```python
from build123d import *

# Parameters (mm, degrees)
SKETCH1_W           = 120
SKETCH1_H           = 92
SKETCH1_R           = 1.5
BOSS_EXTRUDE1_DEPTH = 1
SKETCH2_W           = 1
SKETCH2_H           = 92
BOSS_EXTRUDE2_DEPTH = 23
FILLET1_R           = 3
FILLET2_R           = 3
FILLET3_R           = 3


with BuildPart() as part:
    # Sketch1 → Boss-Extrude1 (new body)
    with BuildSketch(Plane.XY):
        Rectangle(SKETCH1_W, SKETCH1_H)
        with Locations((0, -32)):
            Circle(SKETCH1_R, mode=Mode.SUBTRACT)
        with Locations(Location((0, 32, 0), (0, 0, 180))):
            Circle(SKETCH1_R, mode=Mode.SUBTRACT)
    extrude(amount=BOSS_EXTRUDE1_DEPTH)

    # Sketch2 → Boss-Extrude2 (add)
    with BuildSketch(Plane.XY.offset(1)):
        with Locations((-59.5, 0)):
            Rectangle(SKETCH2_W, SKETCH2_H)
    boss_extrude2 = extrude(amount=BOSS_EXTRUDE2_DEPTH)

    # Fillet1
    fillet1_edges = [part.edges().sort_by_distance(p)[0] for p in [
        (-60, 0, 0),
    ]]
    fillet(fillet1_edges, radius=FILLET1_R)

    # Fillet2
    fillet2_edges = [part.edges().sort_by_distance(p)[0] for p in [
        (-59, 0, 1),
    ]]
    fillet(fillet2_edges, radius=FILLET2_R)

    # Mirror3: Boss-Extrude2 across plane
    add(boss_extrude2.mirror(Plane(origin=(0, 0, 0), x_dir=(0, 0, 1), z_dir=(1, 0, 0))))

    # Fillet3
    fillet3_edges = [part.edges().sort_by_distance(p)[0] for p in [
        (59, 0, 1),
        (60, 0, 0),
    ]]
    fillet(fillet3_edges, radius=FILLET3_R)


solid = part.part
```
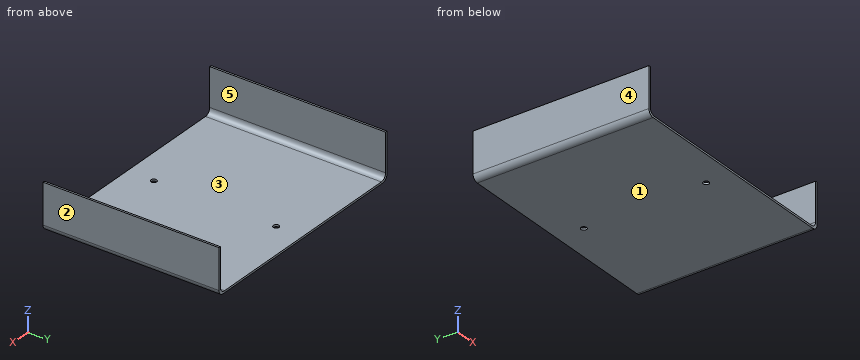
Source: CAD feature listing. Evaluate the final solid. Frame: model axes, mm. Face numbers are marked on the shaded views. A direction names the side the tool comes from. Coordinates: 2 decimals unless noted, no trailing zeros. Loops run counter-clockwise (first coordinate to the right, second up) from the corner with the lowest first, then second, coordinate; pieces in that order, holes last. Notation, with made-up numbers: (56, -33) - (96, -33) arc R23 ccw to (96, 1) - close; hole circle Ø2 at (15, 55). An arc over 180 degrees is marked (long way). Answer as CSV lines item,"result".
1. Ray query, line 1 (Y direction, x = 0, z = 0.6); line 2 (X direction, y = 40.5, z = 7.75); line 3 (Z direction, x = -33.5, y = -24.5). Return the intervals inside material, ascending.
Established:
line 1,"y = -46 to -33.5, -30.5 to 30.5, 33.5 to 46"
line 2,"x = -60 to -59, 59 to 60"
line 3,"z = 0 to 1"
2. Reachability of the marked faces 4 and 5 from +Z, -Z, +X, -X, +Y, -Y: full face, straight path, thin tool, end or side. Return the list, or none.
Established:
face 4,"+Z, -Z, -X, +Y, -Y"
face 5,"+Z, +Y, -Y"
3. Section A-A (y = -32). Return loops of the section in (x, z).
Established:
outline,"(-60, 3) arc R3 ccw to (-57, 0) - (-1.5, 0) - (-1.5, 1) - (-56, 1) arc R3 cw to (-59, 4) - (-59, 24) - (-60, 24) - close; (1.5, 0) - (57, 0) arc R3 ccw to (60, 3) - (60, 24) - (59, 24) - (59, 4) arc R3 cw to (56, 1) - (1.5, 1) - close"
4. Section C-C (z = 13.25). Return loops of the section in (x, y), then the cut area to 3 significant figures.
Established:
outline,"(-60, -46) - (-59, -46) - (-59, 46) - (-60, 46) - close; (59, -46) - (60, -46) - (60, 46) - (59, 46) - close"
area,"184 mm2"
5. Mould query, pull axis X, two halves, no side actions, for the marked faces 1, 2 and 3. Classes: released by +X, released by -X, zero draft, split by the parting line, or undercut.
Established:
face 1,"zero draft"
face 2,"released by +X"
face 3,"undercut"
6. Contact query for flat-ended pins moving along their axis: pin 1 (3.5 mm diameter, centred on x = 0, y = 32, fed in from +Z); pin 2 (2.5 mm diameter, centred on x = 0, y = -32, fed in from +Z). Output: stop coordinate, or through.
Established:
pin 1,"stops at z = 1"
pin 2,"passes through"
7. Section B-B (x = 0). Return loops of the section in (y, z).
Established:
outline,"(-46, 0) - (-33.5, 0) - (-33.5, 1) - (-46, 1) - close; (-30.5, 0) - (30.5, 0) - (30.5, 1) - (-30.5, 1) - close; (33.5, 0) - (46, 0) - (46, 1) - (33.5, 1) - close"
8. Section D-D (y = -12.5). Return loops of the section in (x, z).
Established:
outline,"(-60, 3) arc R3 ccw to (-57, 0) - (57, 0) arc R3 ccw to (60, 3) - (60, 24) - (59, 24) - (59, 4) arc R3 cw to (56, 1) - (-56, 1) arc R3 cw to (-59, 4) - (-59, 24) - (-60, 24) - close"
